Here's how the part is built. I have some questions about the finished solid (model axes, mm). Face numbers are marked on the shaded views. A direction names the side the tool comes from. Round coordinates to 2 decimals unless told otherwise and drop trailing zeros. Write each loop counter-clockwise with the first axis right and the second up, starting at its lowest first coordinate (ties: lowest second). Pieces come first, ordered by that corner, then holes. Notation, with made-up numbers: (34, 85.5) -> (73, 85.5) arc R21 cw to (73, 104.5) -> close; hole circle Ø4 at (13, 64). An arc over 180 degrees is marked (long way). Answer in a Markdown table with one row per item.
from build123d import *

# Parameters (mm, degrees)
F1_DEPTH = 13
F2_R     = 8
F3_R     = 2
F5_DEPTH = 8.73125
F6_R     = 2.25
F7_DEPTH = 13.001
F8_R     = 4
F9_SIZE  = 1.5
F10_SIZE = 0.25


with BuildPart() as f1:
    # F0 (on Top) → F1 (new body)
    with BuildSketch(Plane.XY):
        Polygon((0, 2.747639), (14, 2.747639), (14, 14.747639), (7.071797, 26.747639), (0, 26.747639), (-7.071797, 26.747639), (-14, 14.747639), (-14, 2.747639), align=None)
    extrude(amount=F1_DEPTH)

    # F2
    f2_edges = [f1.edges().sort_by_distance(p)[0] for p in [
        (-14, 14.747639, 6.5),
        (14, 14.747639, 6.5),
    ]]
    fillet(f2_edges, radius=F2_R)

    # F3
    f3_edges = [f1.edges().sort_by_distance(p)[0] for p in [
        (-7.071797, 26.747639, 6.5),
        (7.071797, 26.747639, 6.5),
    ]]
    fillet(f3_edges, radius=F3_R)

    # F4 (on face) → F5 (cut)
    with BuildSketch(Plane.XY.offset(13)):
        with BuildLine():
            Line((-2.54, 26.747639), (-2.54, 18.497639))
            ThreePointArc((-2.54, 18.497639), (0, 15.957639), (2.54, 18.497639))
            Line((2.54, 18.497639), (2.54, 26.747639))
            Line((2.54, 26.747639), (-2.54, 26.747639))
        make_face()
    extrude(amount=-F5_DEPTH, mode=Mode.SUBTRACT)

    # F6 (on face) → F7 (cut, through all)
    with BuildSketch(Plane(origin=(0, 0, 0), x_dir=(1, 0, 0), z_dir=(0, 0, -1))):
        with Locations((-7, -9.497639)):
            Circle(F6_R)
        with Locations((7, -9.497639)):
            Circle(F6_R)
    extrude(amount=-F7_DEPTH, mode=Mode.SUBTRACT)

    # F8
    f8_edges = [f1.edges().sort_by_distance(p)[0] for p in [
        (-14, 2.747639, 6.5),
        (14, 2.747639, 6.5),
    ]]
    fillet(f8_edges, radius=F8_R)

    # F9
    f9_edges = [f1.edges().sort_by_distance(p)[0] for p in [
        (0, 15.957639, 4.26875),
    ]]
    chamfer(f9_edges, length=F9_SIZE)

    # F10
    f10_edges = [f1.edges().sort_by_distance(p)[0] for p in [
        (4.75, 9.497639, 0),
        (-9.25, 9.497639, 0),
        (10.288675, 21.175842, 0),
    ]]
    chamfer(f10_edges, length=F10_SIZE)


solid = f1.part
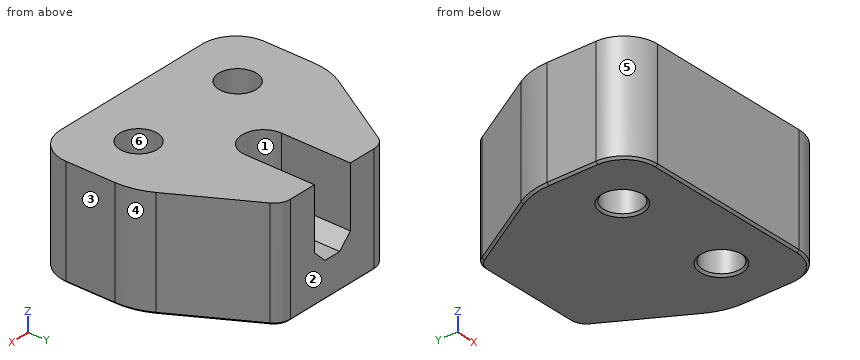
1) For pin 1 (5 mm diameter, centred on y = 21, z = 10, fed in from -X); pin 2 (8 mm diameter, centred on x = -1.5, y = 19.5, fed in from +Z); pin 3 (2 mm diameter, centred on y = 24.5, z = 8, fed in from +X); pin 4 (1 mm diameter, centred on x = 10.5, z = 2.5, fed in from +Y), each with a flat end and sliding along its axis, tell me the tip position at first contact or that it passes through.
Response:
| item | result |
|---|---|
| pin 1 | stops at x = -11.83 |
| pin 2 | stops at z = 13 |
| pin 3 | stops at x = 8.95 |
| pin 4 | stops at y = 21.68 |
2) I need wall thicknesses on line 1 (X direction, y = 11.5, z = 10.25); line 2 (Y direction, x = 7, z = 8.5); line 3 (X direction, y = 12.75, z = 10.5). Which ranges of each line are inside material? Lowest first, please. Write a range as [from, to].
Response:
| item | result |
|---|---|
| line 1 | x = [-14, -8.03], [-5.97, 5.97], [8.03, 14] |
| line 2 | y = [2.75, 7.25], [11.75, 26.43] |
| line 3 | x = [-14, 14] |
3) I want a section at C-C, the plane y = 10.25. Count the separate pieces of the cut face and the enclosed holes in it, and give its area (3 significant figures).
Response:
| item | result |
|---|---|
| separate pieces | 3 |
| enclosed holes | 0 |
| area | 254 mm^2 |
4) I want a section at D-D, the plane y = 20.5. List the corners of the cut face in (x, z) for me.
Response:
| item | result |
|---|---|
| outline | (-10.68, 0.25) -> (-10.39, 0) -> (10.39, 0) -> (10.68, 0.25) -> (10.68, 13) -> (2.54, 13) -> (2.54, 5.77) -> (1.04, 4.27) -> (-1.04, 4.27) -> (-2.54, 5.77) -> (-2.54, 13) -> (-10.68, 13) -> close |
5) I want a section at A-A, the plane z = 2.25. List the corners of the cut face in (x, y) for me.
Response:
| item | result |
|---|---|
| outline | (-14, 6.75) arc R4 ccw to (-10, 2.75) -> (10, 2.75) arc R4 ccw to (14, 6.75) -> (14, 12.6) arc R8 ccw to (12.93, 16.6) -> (7.65, 25.75) arc R2 ccw to (5.92, 26.75) -> (-5.92, 26.75) arc R2 ccw to (-7.65, 25.75) -> (-12.93, 16.6) arc R8 ccw to (-14, 12.6) -> close; hole circle Ø4.5 at (-7, 9.5); hole circle Ø4.5 at (7, 9.5) |
6) We'd pull the mould along Y, two halves only. Please class the marked faces 3, 4, 5 and 6: +Y half, -Y half, draft (parallel to the pull), parting line (faces both ways), or undercut.
Response:
| item | result |
|---|---|
| face 3 | draft |
| face 4 | +Y half |
| face 5 | -Y half |
| face 6 | undercut |
7) I want a section at B-B, the plane x = 0. List the corners of the cut face in (y, z) for me.
Response:
| item | result |
|---|---|
| outline | (2.75, 0.25) -> (3, 0) -> (26.5, 0) -> (26.75, 0.25) -> (26.75, 4.27) -> (17.46, 4.27) -> (15.96, 5.77) -> (15.96, 13) -> (2.75, 13) -> close |
8) Which directions (+Z, -Z, +X, -X, +Y, -Y) give clear straight access to the entire face, cutting with the end or side of a thin tool? Please do the marked faces 1 and 2.
Response:
| item | result |
|---|---|
| face 1 | +Z, +Y |
| face 2 | +Z, -Z, +X, -X, +Y |
